Read the model definition and answer for the solid it produces. Units are mm, in the model's axes. Coordinates: 2 decimals unless noted, no trailing zeros. Write each loop counter-clockwise with the first axis right and the second up, starting at its lowest first coordinate (ties: lowest second). Pieces come first, ordered by that corner, then holes. Notation, with made-up numbers: (60.5, 81.5) -> (115.5, 81.5) arc R22 ccw to (115.5, 87.5) -> close; hole circle Ø7 at (85.25, 24.5). An arc over 180 degrees is marked (long way). Write item = value, one per line. Start each with the question number.
1) Find the intervals of material crossed by line 1 along Y through (x, z) = (-72.6, 20.5) (3 decimals); line 2 along X through (y, z) = (-142.25, 21.25); line 3 along Y through (x, z) = (-73.5, 21) (3 decimals), in increasing order. Write a range as from..to.
2) Section D-D (x = -75) is taken. Determine the outline of the cut face in (y, z) (3 decimals), plus the area to 3 significant figures.
3) Section A-A (x = -72.6) is taken. Determine the outline of the cut face in (y, z) (3 decimals), plus the area to 3 significant figures.
4) Section B-B (y = -144) is taken. Determine the outline of the cut face in (x, z), plus the area to 3 significant figures.
5) Section C-C (z = 18.5) is taken. Determine the outline of the cut face in (x, y) (3 decimals).
from build123d import *

# Parameters (mm, degrees)
BOSS_EXTRUDE1_DEPTH      = 6.35
BOSS_EXTRUDE1_DEPTH_BACK = 6.35
SKETCH1_R                = 2.667
SKETCH2_R                = 10.070680165
SKETCH2_R_2              = 1.905
BOSS_EXTRUDE2_DEPTH      = 16
SKETCH4_W                = 19.172603048
SKETCH4_H                = 6.985
CUT_EXTRUDE2_DEPTH       = 7.62
CUT_EXTRUDE3_DEPTH       = 87.58734866
CUT_EXTRUDE3_DEPTH_BACK  = 87.58734866
SKETCH6_W                = 20.14136033
SKETCH6_H                = 21.08


with BuildPart() as part:
    # Sketch1 → Boss-Extrude1 (new, two sides: drawn at the far end of the back side and taken through both)
    with BuildSketch(Plane.XY.offset(-BOSS_EXTRUDE1_DEPTH_BACK)):
        with Locations((-72.6, -136.95)):
            Circle(SKETCH1_R)
    extrude(amount=BOSS_EXTRUDE1_DEPTH + BOSS_EXTRUDE1_DEPTH_BACK)

    # Sketch2 → Boss-Extrude2 (add)
    with BuildSketch(Plane.XY.offset(6.35)):
        with Locations(Location((-72.6, -142.329319835, 0), (0, 0, 90))):
            Circle(SKETCH2_R)
        with Locations(Location((-72.6, -142.329319835, 0), (0, 0, 90))):
            Circle(SKETCH2_R_2, mode=Mode.SUBTRACT)
    extrude(amount=BOSS_EXTRUDE2_DEPTH)

    # Sketch4 → Cut-Extrude2 (cut)
    with BuildSketch(Plane(origin=(0, 0, 22.35), x_dir=(-1, 0, 0), z_dir=(0, 0, -1))):
        with Locations((72.6, -148.9075)):
            Rectangle(SKETCH4_W, SKETCH4_H)
    extrude(amount=CUT_EXTRUDE2_DEPTH, mode=Mode.SUBTRACT)

    # Sketch6 → Cut-Extrude3 (cut, two sides: drawn at the far end of the back side and taken through both)
    with BuildSketch(Plane.XZ.offset(139.617).offset(-CUT_EXTRUDE3_DEPTH_BACK)):
        with Locations((-72.6, 4.19)):
            Rectangle(SKETCH6_W, SKETCH6_H)
    extrude(amount=CUT_EXTRUDE3_DEPTH + CUT_EXTRUDE3_DEPTH_BACK, mode=Mode.SUBTRACT)


solid = part.part
Answer key:
q1.line_1 = -145.415..-144.234, -140.424..-132.259
q1.line_2 = -82.67..-74.5, -70.7..-62.53
q1.line_3 = -145.415..-144.008, -140.65..-132.299
q2.outline = (-145.415, 14.73) -> (-132.549, 14.73) -> (-132.549, 22.35) -> (-145.415, 22.35) -> close
q2.area = 98.0 mm^2
q3.outline = (-145.415, 14.73) -> (-144.234, 14.73) -> (-144.234, 22.35) -> (-145.415, 22.35) -> close; (-140.424, 14.73) -> (-132.259, 14.73) -> (-132.259, 22.35) -> (-140.424, 22.35) -> close
q3.area = 71.2 mm^2
q4.outline = (-82.53, 14.73) -> (-73.52, 14.73) -> (-73.52, 22.35) -> (-82.53, 22.35) -> close; (-71.68, 14.73) -> (-62.67, 14.73) -> (-62.67, 22.35) -> (-71.68, 22.35) -> close
q4.area = 137 mm^2
q5.outline = (-82.186, -145.415) -> (-63.014, -145.415) arc R10.071 ccw (long way) to start; hole circle Ø3.81 at (-72.6, -142.329)
